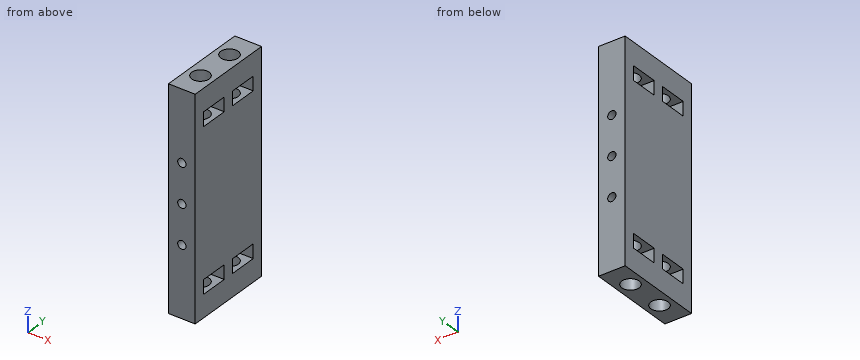
```python
from build123d import *

# Parameters (mm, degrees)
SKETCH1_W               = 9.525
SKETCH1_H               = 32
BOSS_EXTRUDE1_DEPTH     = 77.775
SKETCH2_W               = 5
SKETCH2_H               = 10
NUT_SLOT_DEPTH          = 80.972971997
M6_START                = 9.525
SKETCH3_R               = 3.1
M6_DRILL_DEPTH          = 27
MIRROR2_COPY_1_SKETCH_W = 5
MIRROR2_COPY_1_SKETCH_H = 10
MIRROR2_COPY_1_DEPTH    = 80.972971997
MIRROR2_START           = 9.525
MIRROR2_COPY_2_SKETCH_R = 3.1
MIRROR2_COPY_2_DEPTH    = 27
LPATTERN1_COUNT         = 3
LPATTERN1_PITCH         = 13.8875


with BuildPart() as part:
    # Sketch1 → Boss-Extrude1 (new body)
    with BuildSketch(Plane.XY):
        with Locations((59.5125, 0)):
            Rectangle(SKETCH1_W, SKETCH1_H)
    extrude(amount=BOSS_EXTRUDE1_DEPTH)

    # Sketch2 → Nut Slot (cut, through all)
    with BuildSketch(Plane(origin=(64.275, 0, 0), x_dir=(0, 0, -1), z_dir=(1, 0, 0))):
        with Locations((-67.275, 7)):
            Rectangle(SKETCH2_W, SKETCH2_H)
    nut_slot = extrude(amount=-NUT_SLOT_DEPTH, mode=Mode.SUBTRACT)

    # Sketch3 → M6 Drill (cut)
    with BuildSketch(Plane.XY.offset(77.775).offset(M6_START)):
        with Locations(Location((59.5125, 7, 0), (0, 0, 270))):
            Circle(SKETCH3_R)
    m6_drill = extrude(amount=-M6_DRILL_DEPTH, mode=Mode.SUBTRACT)

    # Mirror1: Nut Slot, M6 Drill across plane
    add(nut_slot.mirror(Plane.ZX), mode=Mode.SUBTRACT)
    add(m6_drill.mirror(Plane.ZX), mode=Mode.SUBTRACT)

    # Mirror2: Nut Slot, M6 Drill across plane
    add(nut_slot.mirror(Plane.XY.offset(38.8875)), mode=Mode.SUBTRACT)
    add(m6_drill.mirror(Plane.XY.offset(38.8875)), mode=Mode.SUBTRACT)

    # Mirror2 copy 1 sketch → Mirror2 copy 1 (cut, through all)
    with BuildSketch(Plane(origin=(64.275, 0, 77.775), x_dir=(0, 0, 1), z_dir=(1, 0, 0))):
        with Locations((-67.275, 7)):
            Rectangle(MIRROR2_COPY_1_SKETCH_W, MIRROR2_COPY_1_SKETCH_H)
    extrude(amount=-MIRROR2_COPY_1_DEPTH, mode=Mode.SUBTRACT)

    # Mirror2 copy 2 sketch → Mirror2 copy 2 (cut)
    with BuildSketch(Plane(origin=(0, 0, 0), x_dir=(1, 0, 0), z_dir=(0, 0, -1)).offset(MIRROR2_START)):
        with Locations(Location((59.5125, 7, 0), (0, 0, 270))):
            Circle(MIRROR2_COPY_2_SKETCH_R)
    extrude(amount=-MIRROR2_COPY_2_DEPTH, mode=Mode.SUBTRACT)

    # Sketch7 → #32 (0.116) Diameter Hole1 (revolve, cut)
    with BuildSketch(Plane(origin=(59.5125, -16, 52.775), x_dir=(0, 0, -1), z_dir=(1, 0, 0))):
        Polygon((0, 0), (0, 10.410187864), (1.4732, 9.525), (1.4732, 0), align=None)
    f_32_0_116_diameter_hole1 = revolve(axis=Axis((59.5125, -22.35, 52.775), (0, 1, 0)), mode=Mode.SUBTRACT)

    # LPattern1: #32 (0.116) Diameter Hole1 ×3
    with Locations(*[(0, 0, -i * LPATTERN1_PITCH) for i in range(1, LPATTERN1_COUNT)]):
        add(f_32_0_116_diameter_hole1, mode=Mode.SUBTRACT)

    # Mirror3: #32 (0.116) Diameter Hole1 across plane
    add(f_32_0_116_diameter_hole1.mirror(Plane.ZX), mode=Mode.SUBTRACT)

    # Mirror3 copy 1 sketch → Mirror3 copy 1 (revolve, cut)
    with BuildSketch(Plane(origin=(59.5125, 16, 38.8875), x_dir=(0, 0, -1), z_dir=(1, 0, 0))):
        Polygon((0, 0), (0, -10.410187864), (1.4732, -9.525), (1.4732, 0), align=None)
    revolve(axis=Axis((59.5125, 22.35, 38.8875), (0, 1, 0)), mode=Mode.SUBTRACT)

    # Mirror3 copy 2 sketch → Mirror3 copy 2 (revolve, cut)
    with BuildSketch(Plane(origin=(59.5125, 16, 25), x_dir=(0, 0, -1), z_dir=(1, 0, 0))):
        Polygon((0, 0), (0, -10.410187864), (1.4732, -9.525), (1.4732, 0), align=None)
    revolve(axis=Axis((59.5125, 22.35, 25), (0, 1, 0)), mode=Mode.SUBTRACT)


solid = part.part
```
Can you work these out from the model? Positions are in its coordinate system, mm. Coordinates: 2 decimals unless noted, no trailing zeros. Loops run counter-clockwise (first coordinate to the right, second up) from the corner with the lowest first, then second, coordinate; pieces in that order, holes last. Notation, with made-up numbers: (10, 16.5) - (50, 16.5) arc R25 cw to (50, 30.5) - close; hole circle Ø3 at (-16, -1.5). An arc over 180 degrees is marked (long way). Use a Markdown table: item, result.
Item 1: I want a section at C-C on y = -7.5. Give the number of separate pieces and of enclosed holes in the cut face, and give its area (3 significant figures).
Numbers:
| item | result |
|---|---|
| separate pieces | 5 |
| enclosed holes | 3 |
| area | 472 mm2 |
Item 2: If I drill on probe 1 along Z at (x, y) = (63.75, 11.5) (3 decimals); probe 2 along Z at (x, y) = (59.5, 11.5) (3 decimals); probe 3 along Y at (x, z) = (63.25, 68), over which ranges is the centre line in solid material (lowest first)? Write a range as from..to.
Numbers:
| item | result |
|---|---|
| probe 1 | z = 0..8, 13..64.775, 69.775..77.775 |
| probe 2 | z = 0..8, 13..23.527, 26.473..37.414, 40.361..51.302, 54.248..64.775, 69.775..77.775 |
| probe 3 | y = -16..-12, -2..2, 12..16 |
Item 3: I want a section at B-B on z = 69. Please give me the cut outline in (x, y) (3 decimals), and give its area (3 significant figures).
Numbers:
| item | result |
|---|---|
| outline | (54.75, -16) - (64.275, -16) - (64.275, -12) - (54.75, -12) - close; (54.75, -2) - (64.275, -2) - (64.275, 2) - (54.75, 2) - close; (54.75, 12) - (64.275, 12) - (64.275, 16) - (54.75, 16) - close |
| area | 114 mm2 |
Item 4: I want a section at A-A on y = 3. Please give me the cut outline in (x, z) (3 decimals), and give its area (3 significant figures).
Numbers:
| item | result |
|---|---|
| outline | (54.75, 0) - (64.275, 0) - (64.275, 8) - (54.75, 8) - close; (54.75, 13) - (64.275, 13) - (64.275, 64.775) - (54.75, 64.775) - close; (54.75, 69.775) - (64.275, 69.775) - (64.275, 77.775) - (54.75, 77.775) - close |
| area | 646 mm2 |
Item 5: Will these pins go through, and if not, where does the flat tip stop? pin 1 (5 mm diameter, centred on x = 59.51, y = 7, fed in from +Z); pin 2 (2.5 mm diameter, centred on x = 59.51, z = 38.89, fed in from -Y); pin 3 (5.5 mm diameter, centred on x = 59.51, y = -7, fed in from -Z) (3 decimals).
Numbers:
| item | result |
|---|---|
| pin 1 | stops at z = 60.3 |
| pin 2 | stops at y = -6.34 |
| pin 3 | stops at z = 17.475 |
